Part model, mm, in its own coordinate system. A direction names the side the tool comes from. Round coordinates to 2 decimals unless told otherwise and drop trailing zeros. Write each loop counter-clockwise with the first axis right and the second up, starting at its lowest first coordinate (ties: lowest second). Pieces come first, ordered by that corner, then holes. Notation, with made-up numbers: M 75,71.5 L 79,71.5 A22 cw 79,105.5 Z; hole C -24.75,-4 d2. An arc over 180 degrees is marked long. Answer as a JSON object with one key per item and string values. Group by question number.
1. Band-saw the part on C-C, the plane x = -24. Write the cut outline in (y, z), plus the area to 3 significant figures.
2. Band-saw the part on D-D, the plane y = -18. Write the cut outline in (x, z).
3. Drill centre lines: line 1 (Z direction, x = 0, y = 3.2); line 2 (Y direction, x = -0.5, z = 3); line 3 (X direction, y = -0.5, z = 5.5). Where is each one in solid material? Low to high. Write a range as from..to.
4. Drop flat-ended pins along their axis: pin 1 (10 mm diameter, centred on x = 8.5, y = 11.5, fed in from +Z); pin 2 (3.5 mm diameter, centred on x = 0, z = 7.02, fed in from +Y); pin 3 (5 mm diameter, centred on y = -9.5, z = 8, fed in from -X); pin 4 (1.5 mm diameter, centred on x = -0.5, y = -1.5, fed in from +Z). Give the stop position or say it passes through.
5. Two-plate mould, pull along Y, no slides. Class faces 3 (the face through (2.769, -5.323, 6.958)), 4 (the face through (-0.321, -4.13, 5.574)), 5 (the face through (1.491, 0, 5)): +Y half, -Y half, draft (parallel to the pull), parting line (faces both ways), or undercut.
6. Which spindle directions (+Z, -Z, +X, -X, +Y, -Y) get a long thin tool onto all of the face, cutting with end or side? Do faces 1 (the face through (-0.02, -2.74, 5.37)), 2 (the face through (-0.321, 4.13, 5.574)). Say none if no direction does.
7. Band-saw the part on A-A, the plane x = 0. Write the cut outline in (y, z).
8. Band-saw the part on B-B, the plane y = 0. Write the cut outline in (x, z).
from build123d import *

# Parameters (mm, degrees)
F0_R          = 30
F1_DEPTH      = 4
F2_R          = 6
F3_DEPTH      = 10
F4_R          = 1.480547
F5_DEPTH      = 25
F5_DEPTH_BACK = 25
F7_DEPTH      = 9.4


with BuildPart() as f1:
    # F0 (on Top) → F1 (new body)
    with BuildSketch(Plane.XY):
        Circle(F0_R)
    extrude(amount=F1_DEPTH)

    # F2 (on Top) → F3 (join)
    with BuildSketch(Plane.XY):
        Circle(F2_R)
    extrude(amount=F3_DEPTH)

    # F4 (on Front) → F5 (cut, two sides)
    with BuildSketch(Plane.XZ) as f5_sk:
        with Locations((0, 7.019453)):
            Circle(F4_R)
    extrude(amount=F5_DEPTH, mode=Mode.SUBTRACT)
    extrude(f5_sk.sketch, amount=-F5_DEPTH_BACK, mode=Mode.SUBTRACT)

    # F6 (on face) → F7 (cut)
    with BuildSketch(Plane.XY.offset(10)):
        with BuildLine():
            Line((-1.491322, 2.3), (-1.491322, -2.3))
            ThreePointArc((-1.491322, -2.3), (0, -2.741175), (1.491322, -2.3))
            Line((1.491322, -2.3), (1.491322, 2.3))
            ThreePointArc((1.491322, 2.3), (0, 2.741175), (-1.491322, 2.3))
        make_face()
    extrude(amount=-F7_DEPTH, mode=Mode.SUBTRACT)


solid = f1.part
Worked answers:
{
 "1": {"outline": "M -18,0 L 18,0 L 18,4 L -18,4 Z", "area": "144 mm^2"},
 "2": {"outline": "M -24,0 L 24,0 L 24,4 L -24,4 Z"},
 "3": {"line 1": "z = 0..5.54, 8.5..10", "line 2": "y = -30..-2.7, 2.7..30", "line 3": "x = -5.98..-1.49, 1.49..5.98"},
 "4": {"pin 1": "stops at z = 4", "pin 2": "stops at y = 6", "pin 3": "passes through", "pin 4": "stops at z = 0.6"},
 "5": {"face 3": "parting line", "face 4": "draft", "face 5": "undercut"},
 "6": {"face 1": "+Z", "face 2": "+Y, -Y"},
 "7": {"outline": "M -30,0 L 30,0 L 30,4 L 6,4 L 6,5.54 L 2.74,5.54 L 2.74,0.6 L -2.74,0.6 L -2.74,5.54 L -6,5.54 L -6,4 L -30,4 Z; M -6,8.5 L -2.74,8.5 L -2.74,10 L -6,10 Z; M 2.74,8.5 L 6,8.5 L 6,10 L 2.74,10 Z"},
 "8": {"outline": "M -30,0 L 30,0 L 30,4 L 6,4 L 6,10 L 1.49,10 L 1.49,0.6 L -1.49,0.6 L -1.49,10 L -6,10 L -6,4 L -30,4 Z"}
}
